For this review, use the dimensioned drawing (mm, ordinates from the lowest corner) and the shaded views. A direction names the side the tool comes from. Give positions to 0.01 mm unless a question says otherwise; leave off trailing zeros. Order: outer loops, then holes, each group sorted by start corner. A loop starts at its lowest first (then second) coordinate and runs counter-clockwise, first axis right, second up. Notation, with made-up numbers: (22, 67) - (27, 67) arc R12 cw to (27, 75) - close; hole circle Ø3 at (37, 16). An arc over 180 degrees is marked (long way). One line per item, written item: value.
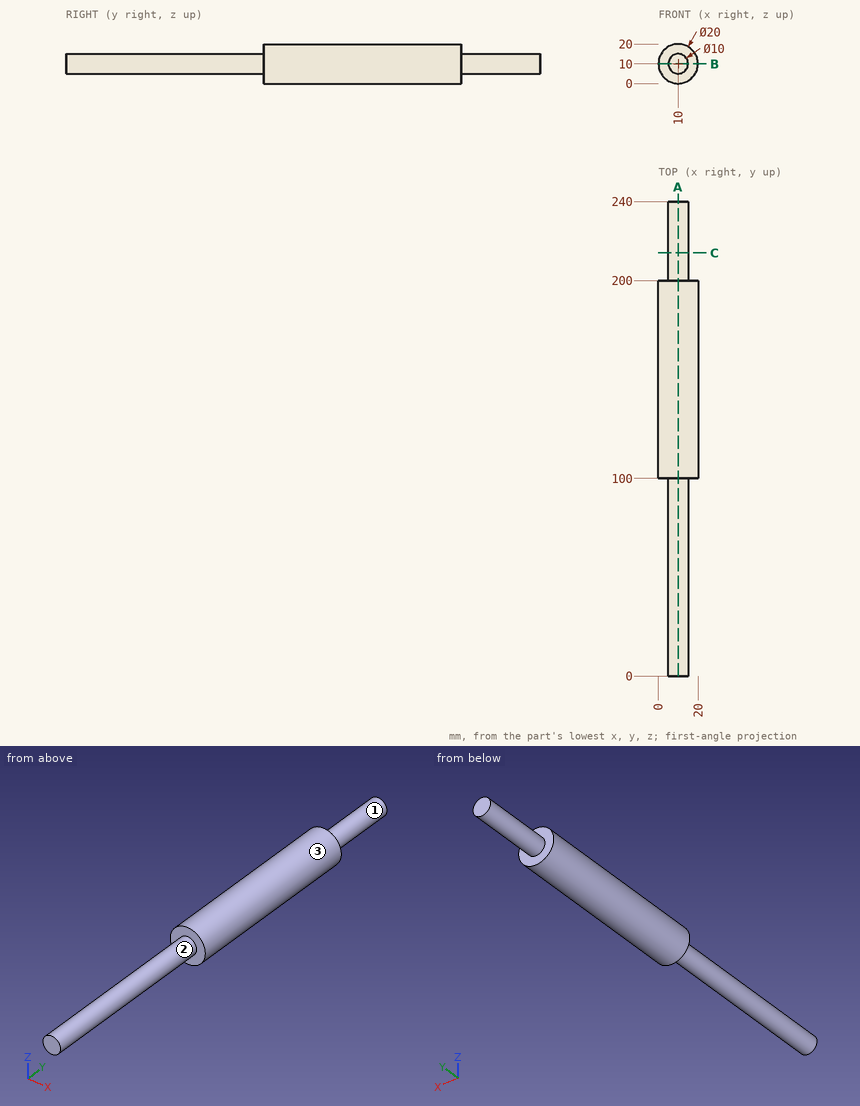
(1) For P1, Ø8, axis at x = 3.5, y = 139, coming from the -Z side; P2, Ø1, axis at x = 16, y = 192.5, coming from the +Z side; P3, Ø2, axis at x = 16, z = 13.5, coming from the +Y side, all flat-tipped, find the tip position at first contact; note any pin that passes through.
Answers below:
P1: stops at z = 0.32
P2: stops at z = 18.35
P3: stops at y = 200
(2) Take a section at B-B (z = 10). Write out the cut boundary in (x, y), then the cut area to 3 significant figures.
Answers below:
outline: (0, 100) - (5, 100) - (5, 0) - (15, 0) - (15, 100) - (20, 100) - (20, 200) - (15, 200) - (15, 240) - (5, 240) - (5, 200) - (0, 200) - close
area: 3,400 mm^2
(3) Take a section at A-A (x = 10). Write out the cut boundary in (y, z).
Answers below:
outline: (0, 5) - (100, 5) - (100, 0) - (200, 0) - (200, 5) - (240, 5) - (240, 15) - (200, 15) - (200, 20) - (100, 20) - (100, 15) - (0, 15) - close
(4) Machinability: for the marked faces 1, 2 and 3, which of the approach directions +Z, -Z, +X, -X, +Y, -Y give a long, thin tool a straight path to every point of the face, cutting with its end or side? Answer none if there is none.
Answers below:
face 1: +Y
face 2: -Y
face 3: +Y, -Y
(5) Take a section at C-C (y = 214). Write out the cut boundary in (x, z).
Answers below:
outline: circle Ø10 at (10, 10)
(6) Wall thickness on line 1 (Y direction, x = 17.5, z = 13.5); line 2 (X direction, y = 219, z = 5.5); line 3 (Z direction, x = 9.75, y = 87): over which ranges is each line inside the solid? List them lowest first. Write a range as from..to.
Answers below:
line 1: y = 100..200
line 2: x = 7.82..12.18
line 3: z = 5.01..14.99
